Answer from the drawing. Dimensions are ordinates in mm from the lowest x, y and z of the part. A direction names the side the tool comes from. Coordinates: 2 decimals unless noted, no trailing zeros. Write each loop counter-clockwise with the first axis right and the second up, starting at its lowest first coordinate (ties: lowest second). Pieces come first, ordered by that corner, then holes. Notation, with made-up numbers: (88, -16.5) -> (117, -16.5) arc R23 ccw to (117, -3.5) -> close; hole circle Ø1 at (38.25, -19). An arc over 180 degrees is marked (long way). One line per item, written item: value. Start each with the question number.
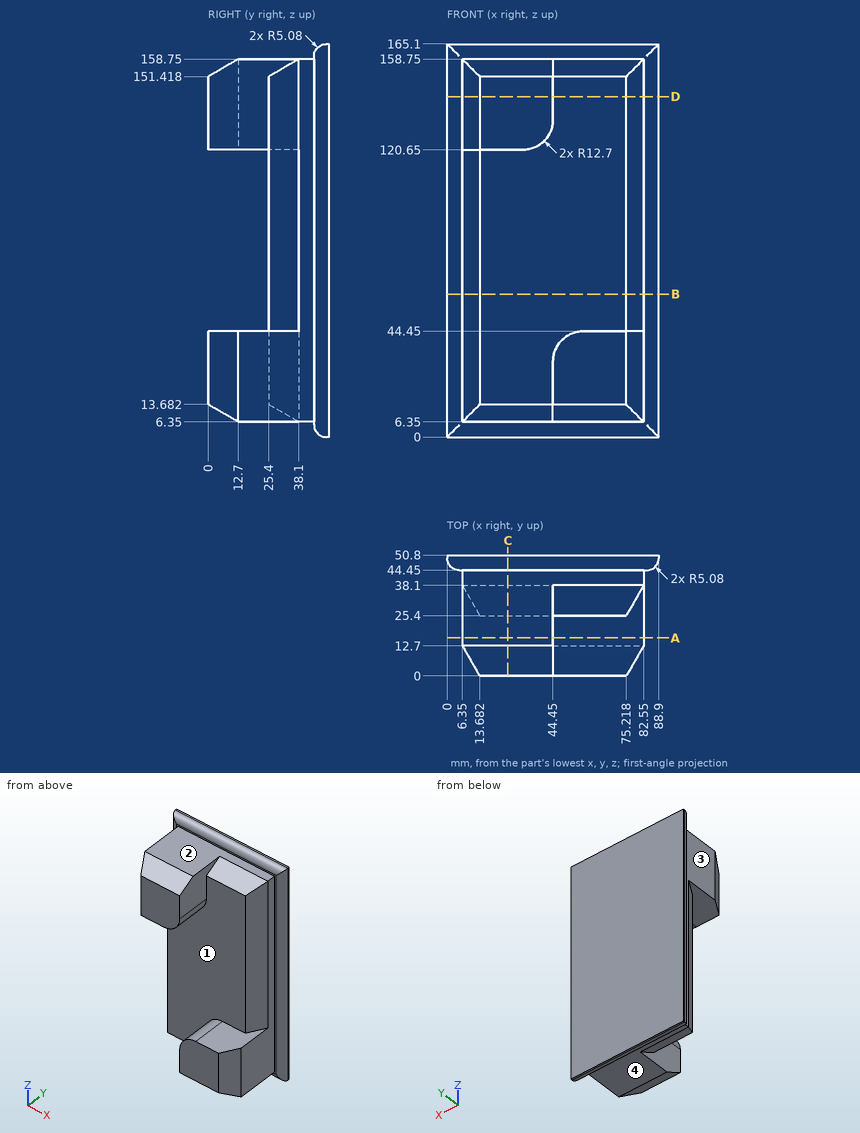
1. A cutting plane is placed at C-C on x = 25.5. Give the vertices of the cut face in (y, z), then the cut area to 4 significant figures.
2. Find the intervals of material crossed by probe 1 along X at (y, z) = (42.5, 21); probe 2 along Z at (x, y) = (6.5, 24.5); probe 3 along Y at (x, z) = (56, 93), in increasing order. Write a range as from..to.
3. A cutting plane is placed at D-D on z = 143. Give the vertices of the cut face in (x, y).
4. A cutting plane is placed at A-A on y = 16. Give the vertices of the cut face in (x, z).
5. Given pin 1 (2 mm diameter, centred on y = 34, z = 95, fed in from +X); pin 2 (1.5 mm diameter, centred on y = 39.5, z = 103, fed in from +X); pin 3 (2 mm diameter, centred on x = 70.5, y = 29, fed in from +Z), each flat-ended and moving along its own axis, determine where each tip first touches the part or whether it passes through.
6. A cutting plane is placed at B-B on z = 60. Give the vertices of the cut face in (x, y), then the cut area to 3 significant figures.
7. A tool of negligible diameter and unlimited length cuts with its end or side. For the marked faces 1, 2, 3 and 4, from which of +Z, -Z, +X, -X, +Y, -Y can it reach the whole face along a straight path? Write none if from no direction.
Derived:
1. outline: (0, 120.65) -> (25.4, 120.65) -> (25.4, 13.68) -> (38.1, 6.35) -> (44.45, 6.35) -> (44.45, 5.08) arc R5.08 ccw to (49.53, 0) -> (50.8, 0) -> (50.8, 165.1) -> (49.53, 165.1) arc R5.08 ccw to (44.45, 160.02) -> (44.45, 158.75) -> (12.7, 158.75) -> (0, 151.42) -> close
1. area: 4,815 mm2
2. probe 1: x = 6.35..82.55
2. probe 2: z = 120.65..158.75
2. probe 3: y = 25.4..50.8
3. outline: (0, 49.53) arc R5.08 ccw to (5.08, 44.45) -> (6.35, 44.45) -> (6.35, 12.7) -> (13.68, 0) -> (44.45, 0) -> (44.45, 25.4) -> (75.22, 25.4) -> (82.55, 38.1) -> (82.55, 44.45) -> (83.82, 44.45) arc R5.08 ccw to (88.9, 49.53) -> (88.9, 50.8) -> (0, 50.8) -> close
4. outline: (6.35, 120.65) -> (31.75, 120.65) arc R12.7 ccw to (44.45, 133.35) -> (44.45, 158.75) -> (6.35, 158.75) -> close; (44.45, 6.35) -> (82.55, 6.35) -> (82.55, 44.45) -> (57.15, 44.45) arc R12.7 ccw to (44.45, 31.75) -> close
5. pin 1: stops at x = 80.76
5. pin 2: stops at x = 82.55
5. pin 3: stops at z = 154.07
6. outline: (0, 49.53) arc R5.08 ccw to (5.08, 44.45) -> (6.35, 44.45) -> (6.35, 38.1) -> (13.68, 25.4) -> (75.22, 25.4) -> (82.55, 38.1) -> (82.55, 44.45) -> (83.82, 44.45) arc R5.08 ccw to (88.9, 49.53) -> (88.9, 50.8) -> (0, 50.8) -> close
6. area: 1,910 mm2
7. face 1: -Y
7. face 2: +Z, +X, -X, -Y
7. face 3: +Z, -Z, -X, -Y
7. face 4: -Z, +X, -X, -Y
